Read the model definition and answer for the solid it produces. Units are mm, in the model's axes. Coordinates: 2 decimals unless noted, no trailing zeros. Loops run counter-clockwise (first coordinate to the right, second up) from the corner with the lowest first, then second, coordinate; pieces in that order, holes last. Notation, with made-up numbers: (73, -11.75) - (105, -11.75) arc R14 cw to (105, 13.25) - close; hole circle Ø10 at (64.5, 8.25). An arc over 180 degrees is marked (long way). Use one line per item in the form item = value.
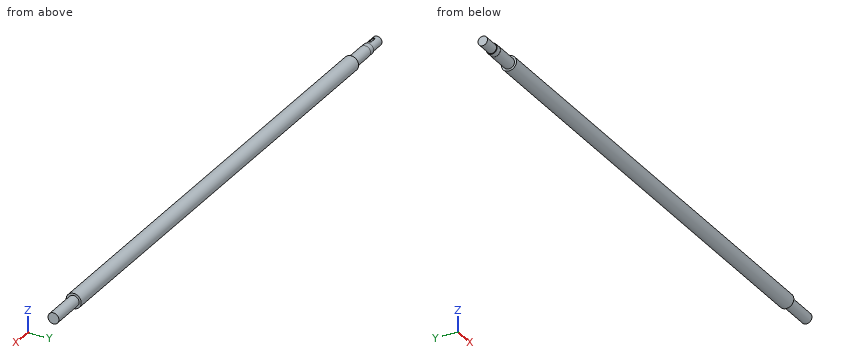
from build123d import *

# Parameters (mm, degrees)
CUT_EXTRUDE_1_DEPTH = 4


with BuildPart() as part:
    # 草图2 → 旋转5 (revolve)
    with BuildSketch(Plane.XY, mode=Mode.PRIVATE) as revolve_5_sk:
        Polygon((0, 0), (0, 17), (58, 17), (58, 19.5), (78, 19.5), (78, 20), (168, 20), (168, 27), (1948, 27), (1948, 19.5), (2078, 19.5), (2078, 0), align=None)
    revolve(revolve_5_sk.sketch.rotate(Axis((41.300309891, 0, 0), (1, 0, 0)), 90), axis=Axis((41.300309891, 0, 0), (1, 0, 0)))

    # 草图3 → 切除-拉伸1 (cut)
    with BuildSketch(Plane.XY.offset(17)):
        with BuildLine():
            Line((20, 2), (40, 2))
            ThreePointArc((40, 2), (45, -3), (40, -8))
            Line((40, -8), (20, -8))
            ThreePointArc((20, -8), (15, -3), (20, 2))
        make_face()
    extrude(amount=-CUT_EXTRUDE_1_DEPTH, mode=Mode.SUBTRACT)


solid = part.part
Item 1: Each of these flat-tipped pins is pushed along its axis until it touches: P1, Ø5, axis at y = 9, z = 5, coming from the -X side; P2, Ø3, axis at x = 396, y = -19.5, coming from the +Z side; P3, Ø4.5, axis at x = 27, z = 15, coming from the -Y side; P4, Ø1, axis at y = 18.5, z = 4, coming from the -X side. Where does it stop, or does it pass through?
Results below:
P1 = 0
P2 = 20.12
P3 = -11.24
P4 = 58
Item 2: Find the intervals of material crossed by L1, parallel to Z at x = 1512.5, y = -2; L2, parallel to Y at x = 1784, z = -4.5; L3, parallel to Y at x = 655, z = -0.5, in increasing order.
Results below:
L1 = -26.93 to 26.93
L2 = -26.62 to 26.62
L3 = -27 to 27
Item 3: The part is cut by section A-A on z = 0. Give the vertices of the cut face in (x, y).
Results below:
outline = (0, -17) - (58, -17) - (58, -19.5) - (78, -19.5) - (78, -20) - (168, -20) - (168, -27) - (1948, -27) - (1948, -19.5) - (2078, -19.5) - (2078, 19.5) - (1948, 19.5) - (1948, 27) - (168, 27) - (168, 20) - (78, 20) - (78, 19.5) - (58, 19.5) - (58, 17) - (0, 17) - close
Item 4: The part is cut by section B-B on x = 1672. Give the vertices of the cut face in (y, z), plus the area to 3 significant figures.
Results below:
outline = circle Ø54 at (0, 0)
area = 2,290 mm²
